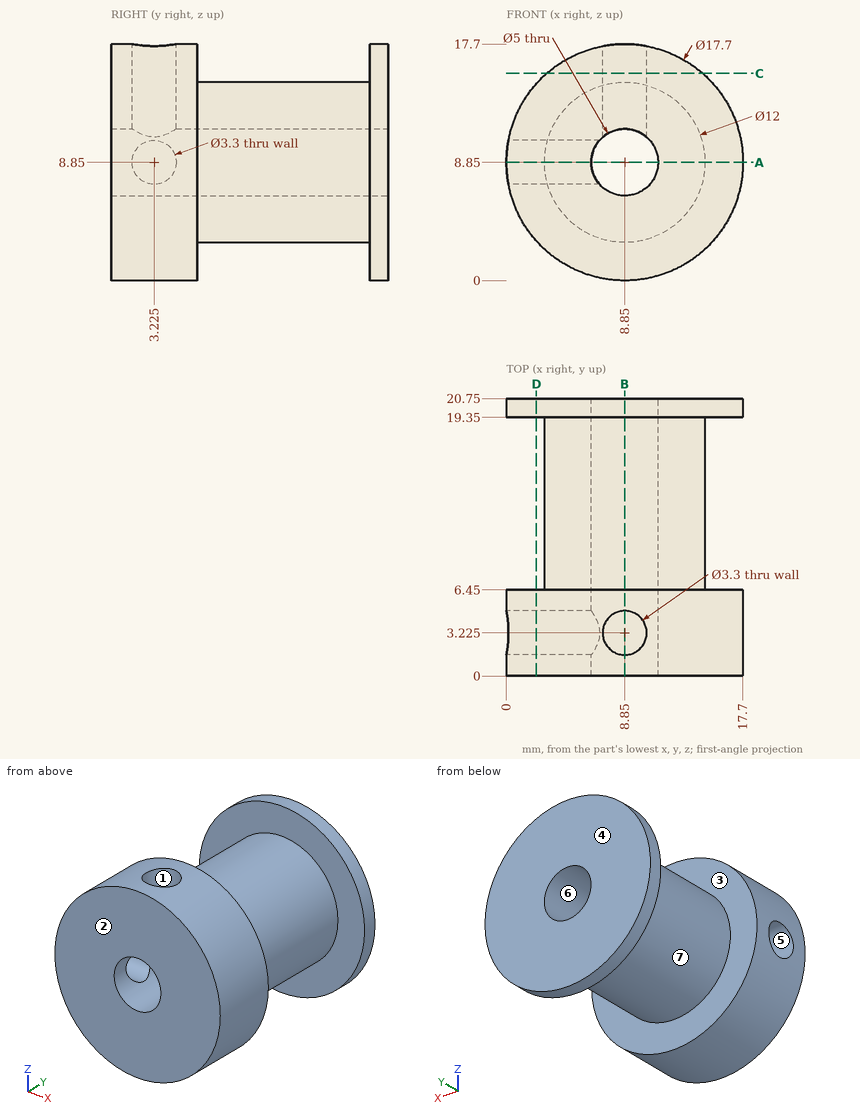
Study the drawing (mm; zero at the part's minimum x, y, z) and answer. A direction names the side the tool comes from. Give positions to 0.01 mm unless a question says otherwise; leave off trailing zeros. Order: outer loops, then holes, each group sorted by start corner. A loop starts at its lowest first (then second) coordinate and runs counter-clockwise, first axis right, second up. Notation, with made-up numbers: (62, 65.25) - (109, 65.25) arc R17 ccw to (109, 76.25) - close; hole circle Ø11 at (89, -26). An arc over 180 degrees is marked (long way). Use one line per item in the form item = value. Start each with the question number.
(1) The mould has two halves that part along Z. Classify the marked faces 4, 5, 6 and 7: released by +Z, released by -Z, zero draft, split by the parting line, or undercut.
(2) Consider line 1 (X direction, y = 8, z = 8.75); line 2 (Y direction, x = 1.5, z = 4.5). Determine where each line is inside the solid, lowest interval first. Write a range as from..to.
(3) A cutting plane is placed at A-A, the plane z = 8.85. Write down the section's boundary in (x, y) (3 decimals), then the cut area to 3 significant figures.
(4) For the marked faces 1, 2 and 3, determine the directions among +Z, -Z, +X, -X, +Y, -Y from which every point of the face is accessible in a straight line to the end or side of a thin tool.
(5) A cutting plane is placed at C-C, the plane z = 15.5. Write down the section's boundary in (x, y) (3 decimals), then the cut area to 3 significant figures.
(6) A cutting plane is placed at D-D, the plane x = 2.25. Write down the section's boundary in (y, z) (3 decimals).
(7) Flat-ended cylindrical pins translate along their axes: pin 1 Ø3 at (x, y) = (9, 2.5) entering from +Z; pin 2 Ø10 at (x, y) = (13.5, 10) entering from -Z; pin 3 Ø4.5 at (x, z) = (8.85, 8.85) entering from +Y; pin 4 Ø4 at (x, y) = (8, 10.5) entering from +Z. Find the tip coordinate at first contact, or state that the pin passes through.
(8) A cutting plane is placed at B-B, the plane x = 8.85. Write down the section's boundary in (y, z) (3 decimals).
Ans:
q1.face_4 = zero draft
q1.face_5 = undercut
q1.face_6 = undercut
q1.face_7 = split by the parting line
q2.line_1 = 2.85..6.35, 11.35..14.85
q2.line_2 = 0..6.45, 19.35..20.75
q3.outline = (0, 0) - (6.35, 0) - (6.35, 1.575) - (0, 1.575) - close; (0, 4.875) - (6.35, 4.875) - (6.35, 20.75) - (0, 20.75) - (0, 19.35) - (2.85, 19.35) - (2.85, 6.45) - (0, 6.45) - close; (11.35, 0) - (17.7, 0) - (17.7, 6.45) - (14.85, 6.45) - (14.85, 19.35) - (17.7, 19.35) - (17.7, 20.75) - (11.35, 20.75) - close
q3.area = 169 mm^2
q4.face_1 = +Z
q4.face_2 = +Z, -Z, +X, -X, -Y
q4.face_3 = none
q5.outline = (3.01, 0) - (14.69, 0) - (14.69, 6.45) - (3.01, 6.45) - close; (3.01, 19.35) - (14.69, 19.35) - (14.69, 20.75) - (3.01, 20.75) - close; hole circle Ø3.3 at (8.85, 3.225)
q5.area = 83.1 mm^2
q6.outline = (0, 2.954) - (6.45, 2.954) - (6.45, 14.746) - (0, 14.746) - close; (19.35, 2.954) - (20.75, 2.954) - (20.75, 14.746) - (19.35, 14.746) - close; hole circle Ø3.3 at (3.225, 8.85)
q7.pin_1 = 17.7
q7.pin_2 = 0.07
q7.pin_3 = through
q7.pin_4 = 14.85
q8.outline = (0, 0) - (6.45, 0) - (6.45, 2.85) - (19.35, 2.85) - (19.35, 0) - (20.75, 0) - (20.75, 6.35) - (0, 6.35) - close; (0, 11.35) - (1.575, 11.35) - (1.575, 17.7) - (0, 17.7) - close; (4.875, 11.35) - (20.75, 11.35) - (20.75, 17.7) - (19.35, 17.7) - (19.35, 14.85) - (6.45, 14.85) - (6.45, 17.7) - (4.875, 17.7) - close
